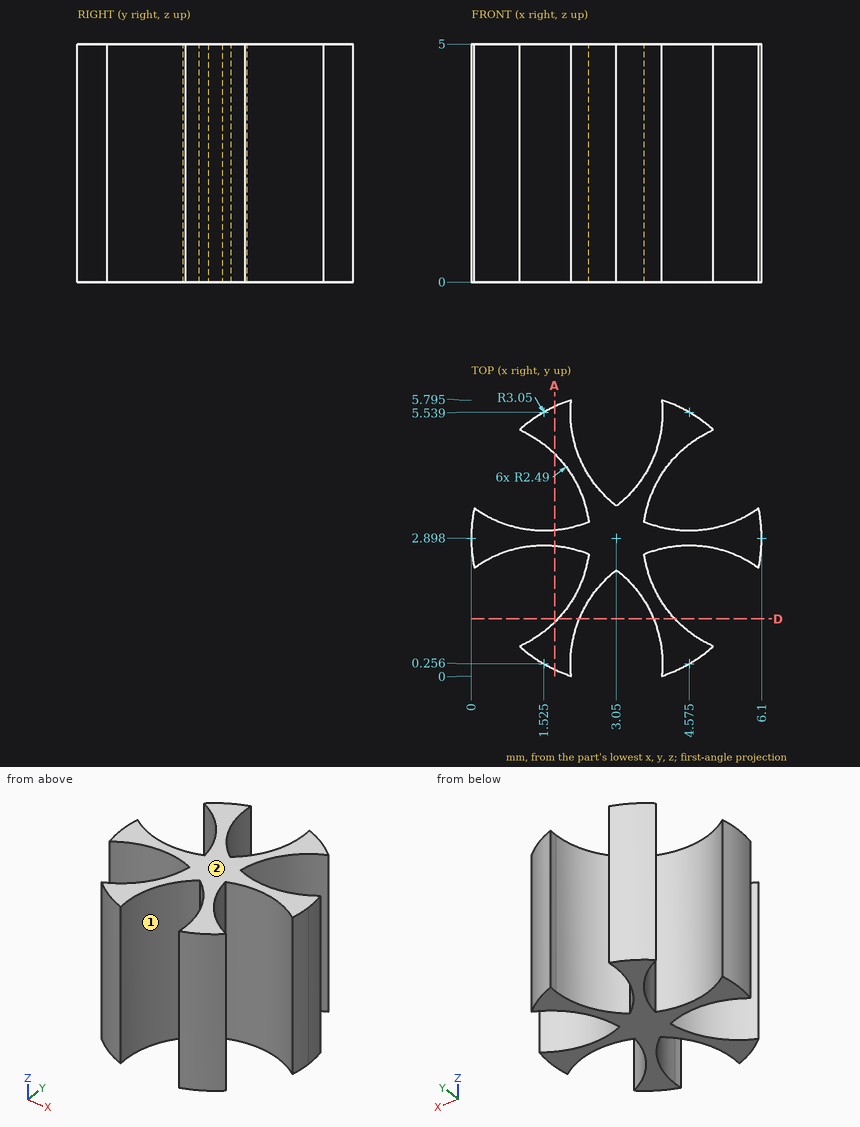
Check sheet for the drawn part. Datum: minimum x, y, z corner. Units: mm. A direction names the side the tool comes from. Give positions to 0.01 mm unless a question says otherwise; leave off trailing zeros. Order: outer loops, then holes, each group sorted by start corner. A loop starts at its lowest first (then second) coordinate and runs counter-clockwise, first axis right, second up. Notation, with made-up numbers: (9, 10.5) -> (39, 10.5) arc R19 cw to (39, 18.5) -> close; hole circle Ø2 at (-37, 70). An arc over 180 degrees is marked (long way). Use a Markdown table: item, result.
1) Tool access check on the marked faces 1 and 2. Record the directions out of +Z, -Z, +X, -X, +Y, -Y that give a thin tool (end or side, any length) a straight path to the whole face; none if there is none.
Results:
| item | result |
|---|---|
| face 1 | +Z, -Z |
| face 2 | +Z, +X, -X, +Y, -Y |
2) Section check A-A, the plane x = 1.75. Record the boundary of the cut face in (y, z), then the cut area to 3 significant figures.
Results:
| item | result |
|---|---|
| outline | (0.14, 0) -> (1.13, 0) -> (1.13, 5) -> (0.14, 5) -> close; (2.74, 0) -> (3.06, 0) -> (3.06, 5) -> (2.74, 5) -> close; (4.67, 0) -> (5.66, 0) -> (5.66, 5) -> (4.67, 5) -> close |
| area | 11.5 mm² |
3) Material ranges on probe 1 along X at (y, z) = (2.5, 2.2) (1 decimal); probe 2 along Y at (x, z) = (1.75, 3.8) (1 decimal); probe 3 along X at (y, z) = (2.1, 2.55), recorded low to high.
Results:
| item | result |
|---|---|
| probe 1 | 0 to 0.4, 2.5 to 3.6, 5.7 to 6.1 |
| probe 2 | 0.1 to 1.1, 2.7 to 3.1, 4.7 to 5.7 |
| probe 3 | 2.36 to 2.9, 3.2 to 3.74 |
4) Depth check by flat-ended pin: pin 1 Ø3 at (x, y) = (5, 2) entering from +Z. Enter the tip coordinate at first touch or a pass-through.
Results:
| item | result |
|---|---|
| pin 1 | z = 5 |
5) Section check D-D, the plane y = 1.2. Record the boundary of the cut face in (x, z).
Results:
| item | result |
|---|---|
| outline | (1.82, 0) -> (2.27, 0) -> (2.27, 5) -> (1.82, 5) -> close; (3.83, 0) -> (4.28, 0) -> (4.28, 5) -> (3.83, 5) -> close |
